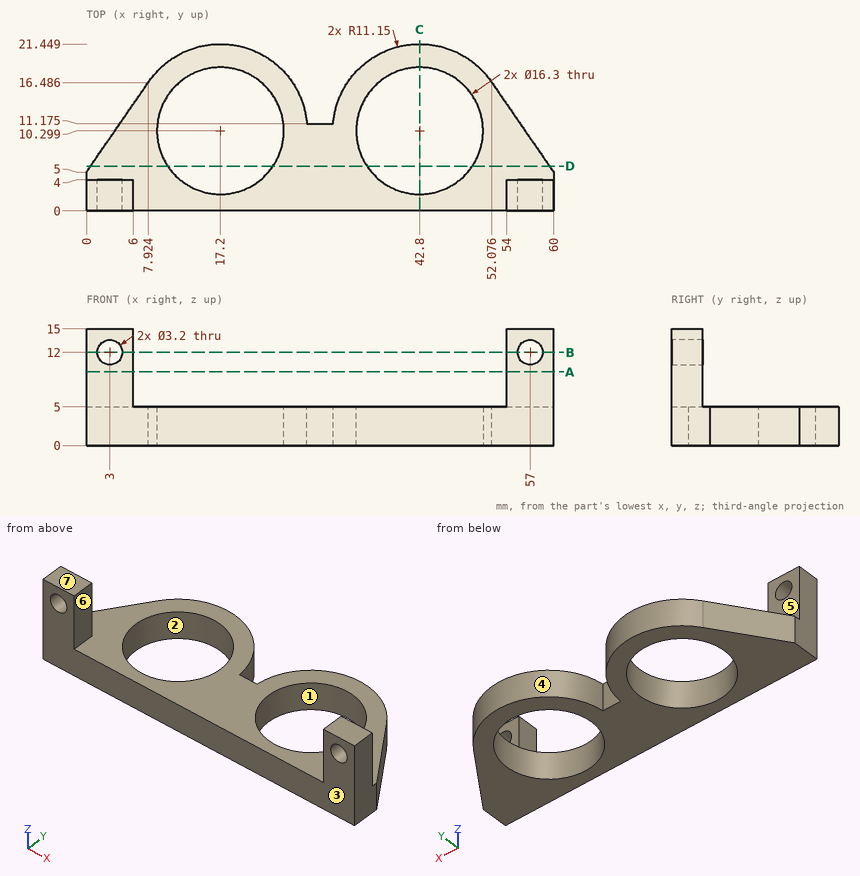
Here's the drawing with two shaded views (mm, measured from the low corner). I have some questions. A direction names the side the tool comes from. Coordinates: 2 decimals unless noted, no trailing zeros. Order: outer loops, then holes, each group sorted by start corner. A loop starts at its lowest first (then second) coordinate and runs counter-clockwise, first axis right, second up.
Q1. Suppose I cut it at B-B on z = 12. Please give me the cut outline in (x, y).
Q2. Suppose I cut it at A-A on z = 9.5. Please give me the cut outline in (x, y), and give its area (3 significant figures).
Q3. Will these pins go through, and if not, where does the flat tip stop? pin 1 (5 mm diameter, centred on x = 2.5, z = 12.5, fed in from +Y); pin 2 (2 mm diameter, centred on x = 28.5, z = 3, fed in from +Y).
Q4. Suppose I cut it at D-D on y = 5.75. Please give me the cut outline in (x, z), and give its area (3 significant figures).
Q5. Suppose I cut it at C-C on x = 42.8. Please give me the cut outline in (y, z).
Q6. Which directions (+Z, -Z, +X, -X, +Y, -Y) give clear straight access to the entire face, cutting with the end or side of a thin tool? Please do the marked faces 5, 6 and 7.
Q7. Please list where these lines run through material, in increasing order: L1, parallel to X at y = 2.85, z = 12; L2, parallel to X at y = 3.5, z = 1 (1 decimal); L3, parallel to X at y = 7.5, z = 2.75 (1 decimal).
Q8. Thinking about a two-plate mould opening in Y: for the marked faces 1, 2, 3 and 4, which applies, released by +Y, released by -Y, zero draft, split by the parting line, or undercut?
Answer:
1. outline: (0, 0) - (1.4, 0) - (1.4, 4) - (0, 4) - close; (4.6, 0) - (6, 0) - (6, 4) - (4.6, 4) - close; (54, 0) - (55.4, 0) - (55.4, 4) - (54, 4) - close; (58.6, 0) - (60, 0) - (60, 4) - (58.6, 4) - close
2. outline: (0, 0) - (6, 0) - (6, 4) - (0, 4) - close; (54, 0) - (60, 0) - (60, 4) - (54, 4) - close
2. area: 48.0 mm2
3. pin 1: stops at y = 4
3. pin 2: stops at y = 14.57
4. outline: (0.52, 0) - (10.44, 0) - (10.44, 5) - (0.52, 5) - close; (23.96, 0) - (36.04, 0) - (36.04, 5) - (23.96, 5) - close; (49.56, 0) - (59.48, 0) - (59.48, 5) - (49.56, 5) - close
4. area: 160 mm2
5. outline: (0, 0) - (2.15, 0) - (2.15, 5) - (0, 5) - close; (18.45, 0) - (21.45, 0) - (21.45, 5) - (18.45, 5) - close
6. face 5: +Z, +X, -X, +Y
6. face 6: +Z, +Y, -Y
6. face 7: +Z, +X, -X, +Y, -Y
7. L1: x = 0 to 1.4, 4.6 to 6, 54 to 55.4, 58.6 to 60
7. L2: x = 0 to 12.7, 21.7 to 38.3, 47.3 to 60
7. L3: x = 1.7 to 9.5, 24.9 to 35.1, 50.5 to 58.3
8. face 1: undercut
8. face 2: undercut
8. face 3: released by -Y
8. face 4: released by +Y
